```python
from build123d import *

# Parameters (mm, degrees)
F0_W          = 249.936
F0_H          = 359.918
F1_DEPTH      = 127
F2_T          = -2.54
F3_W          = 14.986
F3_H          = 50.8
F4_DEPTH      = 73.152
F5_R          = 6.731
F6_DEPTH      = 127.001
F6_DEPTH_BACK = 127.001
F7_R          = 3.175
F8_DEPTH      = 2.54
F9_R          = 4.064
F10_DEPTH     = 75.693
F11_W         = 3.81
F11_H         = 359.918
F12_DEPTH     = 139.7
F14_DEPTH     = 163.831


with BuildPart() as f1:
    # F0 (on Right) → F1 (new body, symmetric)
    with BuildSketch(Plane.YZ):
        Rectangle(F0_W, F0_H)
    extrude(amount=F1_DEPTH, both=True)

    # F2
    f2_openings = [f1.faces().sort_by_distance(p)[0] for p in [
        (0, -124.968, 0),
    ]]
    offset(amount=F2_T, openings=f2_openings)

    # F3 (on face) → F4 (join)
    with BuildSketch(Plane(origin=(0, 124.968, 0), x_dir=(-1, 0, 0), z_dir=(0, 1, 0))):
        with Locations((69.85, -94.361)):
            Rectangle(F3_W, F3_H)
        with Locations((69.85, 58.039)):
            Rectangle(F3_W, F3_H)
        with Locations((0, -94.361)):
            Rectangle(F3_W, F3_H)
        with Locations((0, 58.039)):
            Rectangle(F3_W, F3_H)
        with Locations((-69.85, -94.361)):
            Rectangle(F3_W, F3_H)
        with Locations((-69.85, 58.039)):
            Rectangle(F3_W, F3_H)
    extrude(amount=F4_DEPTH)

    # F5 (on Right) → F6 (cut, two sides)
    with BuildSketch(Plane.YZ) as f6_sk:
        with Locations((185.674, 71.501)):
            Circle(F5_R)
        with Locations((185.674, 44.577)):
            Circle(F5_R)
        with Locations((185.674, -80.899)):
            Circle(F5_R)
        with Locations((185.674, -107.823)):
            Circle(F5_R)
    extrude(amount=F6_DEPTH, mode=Mode.SUBTRACT)
    extrude(f6_sk.sketch, amount=-F6_DEPTH_BACK, mode=Mode.SUBTRACT)

    # F7 (on face) → F8 (cut, through all)
    with BuildSketch(Plane(origin=(0, 0, -179.959), x_dir=(1, 0, 0), z_dir=(0, 0, -1))):
        with Locations((-109.22, 72.136)):
            Circle(F7_R)
        with Locations((109.22, 72.136)):
            Circle(F7_R)
        with Locations((95.25, -40.132)):
            Circle(F7_R)
        with Locations((-95.25, -40.132)):
            Circle(F7_R)
    extrude(amount=-F8_DEPTH, mode=Mode.SUBTRACT)

    # F9 (on face) → F10 (cut, through all)
    with BuildSketch(Plane.XZ.offset(-122.428)):
        with Locations((-114.3, 77.089)):
            Circle(F9_R)
        with Locations((114.3, 77.089)):
            Circle(F9_R)
        with Locations((114.3, -113.411)):
            Circle(F9_R)
        with Locations((-114.3, -113.411)):
            Circle(F9_R)
    extrude(amount=-F10_DEPTH, mode=Mode.SUBTRACT)

    # F11 (on face) → F12 (join)
    with BuildSketch(Plane(origin=(0, 124.968, 0), x_dir=(-1, 0, 0), z_dir=(0, 1, 0))):
        with Locations((-34.925, 0)):
            Rectangle(F11_W, F11_H)
        with Locations((34.925, 0)):
            Rectangle(F11_W, F11_H)
    extrude(amount=F12_DEPTH)

    # F13 (on face) → F14 (cut, through all)
    with BuildSketch(Plane.YZ.offset(36.83)):
        Polygon((264.668, 103.759), (264.668, 179.959), (188.468, 179.959), (239.268, 129.159), (239.268, -179.959), (264.668, -179.959), align=None)
    extrude(amount=-F14_DEPTH, mode=Mode.SUBTRACT)


solid = f1.part
```
Design review of the part built by this model. Coordinates are the model's own, in mm. A direction names the side the tool comes from. Coordinates: 2 decimals unless noted, no trailing zeros. Loops run counter-clockwise (first coordinate to the right, second up) from the corner with the lowest first, then second, coordinate; pieces in that order, holes last.
Q1. We need section A-A on y = 70. State the section outline as (x, z) points, and give its area (3 significant figures).
Reported:
outline: (-127, -179.96) - (127, -179.96) - (127, 179.96) - (-127, 179.96) - close; hole (-124.46, -177.42) - (124.46, -177.42) - (124.46, 177.42) - (-124.46, 177.42) - close
area: 3,090 mm2
Q2. For pin 1 (7.5 mm diameter, centred on x = -73, y = 147, fed in from +Z); pin 2 (3 mm diameter, centred on x = -34.5, z = 130.5, fed in from -Y); pin 3 (21.5 mm diameter, centred on y = 185.674, z = 71.501, fed in from +X), all flat-tipped, find the tip position at first contact; note any pin that passes through.
Reported:
pin 1: stops at z = 83.44
pin 2: stops at y = 122.43
pin 3: stops at x = 77.34
Q3. The part is to be moulded in two halves that separate along Z. For faces 1 (the face through (2, -26, -179.959)), 2 (the face through (69.745, 184.798, 78.175)), 3 (the face through (124.46, -3, 2)), 4 (the face through (-70, 198.12, 58)), say which applies: +Z half, -Z half, draft (parallel to the pull), parting line (faces both ways), or undercut.
Reported:
face 1: -Z half
face 2: undercut
face 3: undercut
face 4: draft
Q4. We need section C-C on x = -19.5. State the section outline as (y, z) points.
Reported:
outline: (-124.97, -179.96) - (124.97, -179.96) - (124.97, 179.96) - (-124.97, 179.96) - (-124.97, 177.42) - (122.43, 177.42) - (122.43, -177.42) - (-124.97, -177.42) - close
Q5. We need section B-B on z = 109. State the section outline as (x, y) points.
Reported:
outline: (-127, -124.97) - (-124.46, -124.97) - (-124.46, 122.43) - (124.46, 122.43) - (124.46, -124.97) - (127, -124.97) - (127, 124.97) - (36.83, 124.97) - (36.83, 239.27) - (33.02, 239.27) - (33.02, 124.97) - (-33.02, 124.97) - (-33.02, 239.27) - (-36.83, 239.27) - (-36.83, 124.97) - (-127, 124.97) - close
Q6. Tool access review of faces 5 (the face through (77.343, 161, 58)), 6 (the face through (2, -3, -177.419)), 7 (the face through (-70, 198.12, -94)), 8 (the face through (-69.75, 184.8, 51.25)): name each direction out of +Z, -Z, +X, -X, +Y, -Y from which nothing blocks a thin tool from reaching the whole face with its end or side.
Reported:
face 5: +Z, -Z, +X, +Y
face 6: -Y
face 7: +Z, -Z, -X, +Y
face 8: -X
Q7. To check wall thickness, follow line 1 (Z direction, x = 114.3, y = 123.4) (3 decimals); line 2 (X direction, y = 142, z = 77); line 3 (X direction, y = 205, z = 118). State the ranges of each line that lie inside material, in increasing order.
Reported:
line 1: z = -179.959 to -117.475, -109.347 to 73.025, 81.153 to 179.959
line 2: x = -77.34 to -62.36, -36.83 to -33.02, -7.49 to 7.49, 33.02 to 36.83, 62.36 to 77.34
line 3: x = -36.83 to -33.02, 33.02 to 36.83
